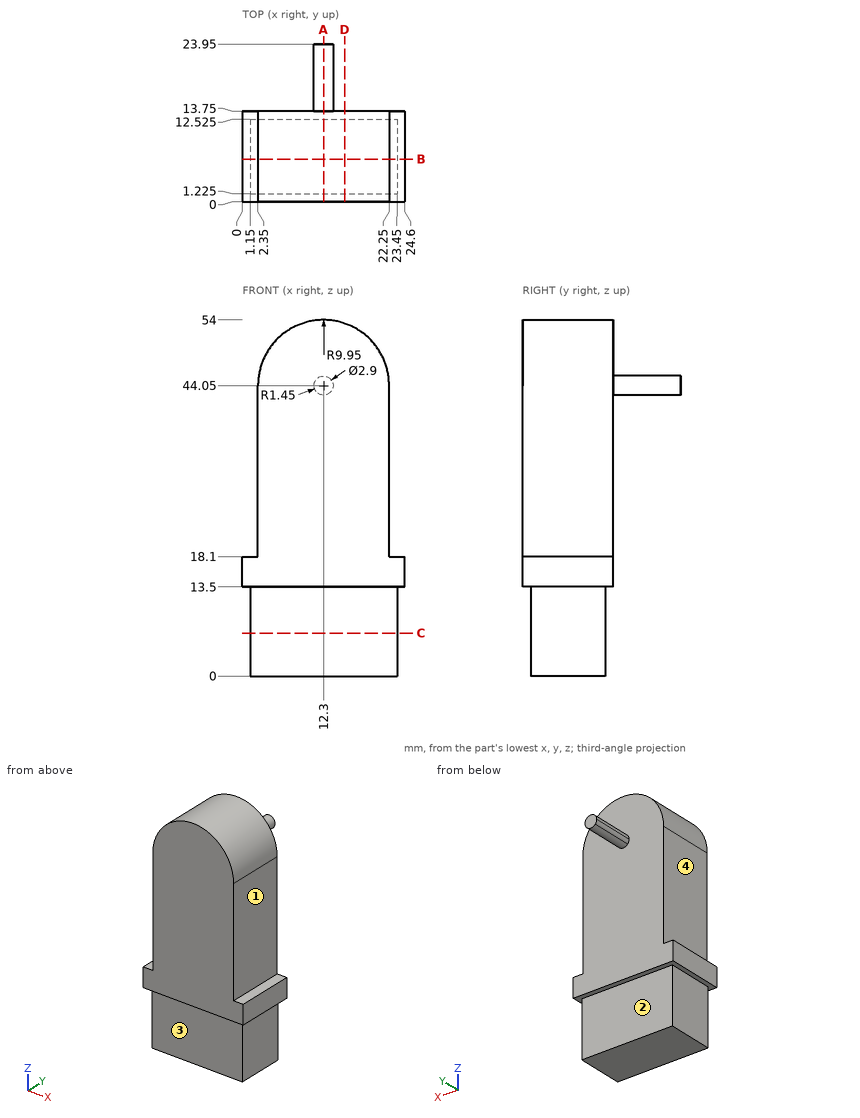
Geometry check sheet. Reference: drawing and pictorial views, mm from the part's lowest x, y, z. A direction names the side the tool comes from. Round coordinates to 2 decimals unless told otherwise and drop trailing zeros. Loops run counter-clockwise (first coordinate to the right, second up) from the corner with the lowest first, then second, coordinate; pieces in that order, holes last. Notation, with made-up numbers: M 18.5,14 L 73.5,14 A21 ccw 73.5,27 Z; hole C 88,60 d3. An arc over 180 degrees is marked long. One line per item, written item: value.
(1) Thickness scan on line 1 (Y direction, x = 10, z = 15); line 2 (X direction, y = 8.5, z = 41); line 3 (Z direction, x = 23.75, y = 7.25). Record the ranges inside material, lowest first.
Computed values:
line 1: y = 0 to 13.75
line 2: x = 2.35 to 22.25
line 3: z = 13.5 to 18.1
(2) Sectioned sample at B-B, the plane y = 6.5. Record the cut outline in (x, z).
Computed values:
outline: M 0,13.5 L 1.15,13.5 L 1.15,0 L 23.45,0 L 23.45,13.5 L 24.6,13.5 L 24.6,18.1 L 22.25,18.1 L 22.25,44.05 A9.95 ccw 2.35,44.05 L 2.35,18.1 L 0,18.1 Z
(3) Sectioned sample at A-A, the plane x = 12.3. Record the cut outline in (y, z) (3 decimals), then the cut area to 3 significant figures.
Computed values:
outline: M 0,13.5 L 1.225,13.5 L 1.225,0 L 12.525,0 L 12.525,13.5 L 13.75,13.5 L 13.75,42.6 L 23.95,42.6 L 23.95,45.5 L 13.75,45.5 L 13.75,54 L 0,54 Z
area: 739 mm^2
(4) Depth check by flat-ended pin: pin 1 Ø7 at (x, z) = (17, 4) entering from +Y (3 decimals); pin 2 Ø7.5 at (x, z) = (11, 32) entering from +Y; pin 3 Ø0.7 at (x, y) = (1.5, 5.5) entering from +Z. Enter the tip coordinate at first touch or a pass-through.
Computed values:
pin 1: stops at y = 12.525
pin 2: stops at y = 13.75
pin 3: stops at z = 18.1
(5) Access from +Z, -Z, +X, -X, +Y, -Y to the whole of each face (thin tool, end or side, straight path). Record for the marked faces 1, 2, 3 and 4.
Computed values:
face 1: +Z, +X, +Y, -Y
face 2: -Z, +X, -X, +Y
face 3: -Z, +X, -X, -Y
face 4: +Z, -X, +Y, -Y
(6) Sectioned sample at C-C, the plane z = 6.5. Record the cut outline in (x, y) (3 decimals), then the cut area to 3 significant figures.
Computed values:
outline: M 1.15,1.225 L 23.45,1.225 L 23.45,12.525 L 1.15,12.525 Z
area: 252 mm^2
(7) Sectioned sample at D-D, the plane x = 15.5. Record the cut outline in (y, z) (3 decimals), then the cut area to 3 significant figures.
Computed values:
outline: M 0,13.5 L 1.225,13.5 L 1.225,0 L 12.525,0 L 12.525,13.5 L 13.75,13.5 L 13.75,53.471 L 0,53.471 Z
area: 702 mm^2
